from build123d import *

# Parameters (mm, degrees)
F1_DEPTH  = 220
F2_W      = 5
F2_H      = 5
F3_DEPTH  = 885
F4_W      = 650
F4_H      = 5
F5_DEPTH  = 5
F6_W      = 5
F6_H      = 5
F7_DEPTH  = 285
F8_R      = 15
F9_DEPTH  = 800
F10_R     = 2.5
F11_DEPTH = 25
F12_R     = 2.5
F13_DEPTH = 25


with BuildPart() as f1:
    # F0 (on Top) → F1 (new body)
    with BuildSketch(Plane.XY):
        Polygon((-345, -450), (-325, -450), (-325, -430), (-325, 430), (325, 430), (325, 150), (345, 150), (345, 450), (-345, 450), align=None)
    extrude(amount=F1_DEPTH)

    # F2 (on face) → F3 (cut)
    with BuildSketch(Plane.XZ.offset(450)):
        with Locations((-327.5, 192.5)):
            Rectangle(F2_W, F2_H)
    extrude(amount=-F3_DEPTH, mode=Mode.SUBTRACT)

    # F4 (on face) → F5 (cut)
    with BuildSketch(Plane.XZ.offset(-430)):
        with Locations((0, 192.5)):
            Rectangle(F4_W, F4_H)
    extrude(amount=-F5_DEPTH, mode=Mode.SUBTRACT)

    # F6 (on face) → F7 (cut)
    with BuildSketch(Plane.XZ.offset(-150)):
        with Locations((327.5, 192.5)):
            Rectangle(F6_W, F6_H)
    extrude(amount=-F7_DEPTH, mode=Mode.SUBTRACT)

    # F8 (on face) → F9 (cut)
    with BuildSketch(Plane.YZ.offset(345)):
        with Locations((190, 120)):
            Circle(F8_R)
    extrude(amount=-F9_DEPTH, mode=Mode.SUBTRACT)

    # F10 (on face) → F11 (cut)
    with BuildSketch(Plane.YZ.offset(-325)):
        with Locations((-300, 150)):
            Circle(F10_R)
        with Locations((-150, 150)):
            Circle(F10_R)
        with Locations((0, 150)):
            Circle(F10_R)
        with Locations((150, 150)):
            Circle(F10_R)
        with Locations((300, 150)):
            Circle(F10_R)
    extrude(amount=-F11_DEPTH, mode=Mode.SUBTRACT)

    # F12 (on face) → F13 (cut)
    with BuildSketch(Plane.XZ.offset(-430)):
        with Locations((-172.5, 150)):
            Circle(F12_R)
        with Locations((-22.5, 150)):
            Circle(F12_R)
        with Locations((127.5, 150)):
            Circle(F12_R)
    extrude(amount=-F13_DEPTH, mode=Mode.SUBTRACT)


solid = f1.part
Geometry check sheet. Reference: the model listing, model coordinates, mm. A direction names the side the tool comes from. Round coordinates to 2 decimals unless told otherwise and drop trailing zeros. Write each loop counter-clockwise with the first axis right and the second up, starting at its lowest first coordinate (ties: lowest second). Pieces come first, ordered by that corner, then holes. Notation, with made-up numbers: (-22, 6) - (21, 6) arc R12 cw to (21, 28) - close; hole circle Ø8 at (89.5, 6.5). An arc over 180 degrees is marked (long way). One line per item, written item: value.
1. Mould release check, pull along X, two halves, no side actions. Record for faces 1 (the face through (-325, -16, 94)), 2 (the face through (-335, -450, 108)), 3 (the face through (345, 298, 108)): released by +X, released by -X, zero draft, split by the parting line, or undercut.
The answers:
face 1: undercut
face 2: zero draft
face 3: released by +X
2. Depth check by flat-ended pin: pin 1 Ø3 at (x, z) = (275.5, 87.5) entering from -Y; pin 2 Ø3 at (x, z) = (127.5, 150) entering from -Y; pin 3 Ø2.5 at (y, z) = (-211, 192.5) entering from +X. Enter the tip coordinate at first touch or a pass-through.
The answers:
pin 1: stops at y = 430
pin 2: passes through
pin 3: stops at x = -330
3. Cross-section at A-A on z = 120. Record the boundary of the cut face in (x, y), and give its area (3 significant figures).
The answers:
outline: (-345, -450) - (-325, -450) - (-325, 175) - (-345, 175) - close; (-345, 205) - (-325, 205) - (-325, 430) - (325, 430) - (325, 205) - (345, 205) - (345, 450) - (-345, 450) - close; (325, 150) - (345, 150) - (345, 175) - (325, 175) - close
area: 35,800 mm^2
4. Cross-section at D-D on z = 178. Record the boundary of the cut face in (x, y).
The answers:
outline: (-345, -450) - (-325, -450) - (-325, 430) - (325, 430) - (325, 150) - (345, 150) - (345, 450) - (-345, 450) - close
5. Cross-section at C-C on y = 333. Record the boundary of the cut face in (x, z), and give its area (3 significant figures).
The answers:
outline: (-345, 0) - (-325, 0) - (-325, 190) - (-330, 190) - (-330, 195) - (-325, 195) - (-325, 220) - (-345, 220) - close; (325, 0) - (345, 0) - (345, 220) - (325, 220) - (325, 195) - (330, 195) - (330, 190) - (325, 190) - close
area: 8,750 mm^2
6. Cross-section at B-B on y = 190. Record the boundary of the cut face in (x, z).
The answers:
outline: (-345, 0) - (-325, 0) - (-325, 105) - (-345, 105) - close; (-345, 135) - (-325, 135) - (-325, 190) - (-330, 190) - (-330, 195) - (-325, 195) - (-325, 220) - (-345, 220) - close; (325, 0) - (345, 0) - (345, 105) - (325, 105) - close; (325, 135) - (345, 135) - (345, 220) - (325, 220) - (325, 195) - (330, 195) - (330, 190) - (325, 190) - close
7. Set-up check for faces 4 (the face through (5, 450, 108)), 5 (the face through (335, 150, 108)), 6 (the face through (-5, 430, 94)): record each of +Z, -Z, +X, -X, +Y, -Y from which the full face is reachable in a straight line by a thin tool's end or side.
The answers:
face 4: +Z, -Z, +X, -X, +Y
face 5: +Z, -Z, +X, -Y
face 6: +Z, -Z, -Y
8. Scan lines: L1, parallel to X at y = 439.25, z = 150; L2, parallel to Y at x = -338, z = 150; L3, parallel to X at y = 362, z = 20. Record each from-to range of solid material in increasing order.
The answers:
L1: x = -345 to -175, -170 to -25, -20 to 125, 130 to 345
L2: y = -450 to -302.5, -297.5 to -152.5, -147.5 to -2.5, 2.5 to 147.5, 152.5 to 297.5, 302.5 to 450
L3: x = -345 to -325, 325 to 345
